Autodesk Inventor part; units mm, degrees
ref_plane "YZ Plane" through (0, 0, 0) normal (1, 0, 0) x (0, 1, 0)
ref_plane "XZ Plane" through (0, 0, 0) normal (0, 1, 0) x (-1, 0, 0)
ref_plane "XY Plane" through (0, 0, 0) normal (0, 0, 1) x (1, 0, 0)
sketch "Sketch1" plane through (0, 0, 0) normal (0, 0, 1) x (1, 0, 0)
  line L0 (0, 0) -> (9.525, 0)
  line L1 (9.525, 0) -> (9.525, 38.1)
  line L2 (9.525, 38.1) -> (31.75, 38.1)
  line L3 (0, 0) -> (0, 63.5) construction
  line L4 (0, 63.5) -> (-3.175, 63.5) construction
  line L5 (-3.175, 63.5) -> (31.75, 38.1)
  line L6 (0, 0) -> (0, 31.75)
  line L7 (4.7625, 0) -> (4.7625, 100.076) construction
  arc A0 (0, 31.75) -> (-3.175, 63.5) centre (-18.6849, 45.9153) ccw
  dimension "d0" = 9.525
  dimension "d1" = 38.1
  dimension "d2" = 22.225
  dimension "d3" = 63.5
  dimension "d4" = 3.175
  dimension "d5" = 4.7625
extrude "Extrusion1" add sketch "Sketch1" along normal blind 12.7
sketch "Sketch2" plane through (9.525, 0, 0) normal (1, 0, 0) x (0, 0, -1)
  line L0 (0, 0) -> (0, 38.1)
  line L1 (0, 0) -> (-12.7, 0)
  circle A0 centre (-6.35, 7.62) radius 3.3782
  circle A1 centre (-3.9688, 25.4) radius 1.5875
  circle A2 centre (-8.7312, 17.4625) radius 1.5875
  dimension "d8" = 6.7564
  dimension "d10" = 6.35
  dimension "d11" = 7.62
  dimension "d12" = 3.175
  dimension "d13" = 3.175
  dimension "d15" = 4.7625
  dimension "d16" = 3.9688
  dimension "d17" = 25.4
  dimension "d24" = 7.9375
extrude "Extrusion2" cut sketch "Sketch2" against normal blind 12.7
fillet "Fillet1" radius 3.175 1 edges at (9.525, 38.1, 6.35)
fillet "Fillet2" radius 0.3175 1 edges at (-3.175, 63.5, 6.35)
fillet "Fillet3" radius 0.3175 1 edges at (0, 31.75, 6.35)
fillet "Fillet4" radius 0.3175 1 edges at (31.75, 38.1, 6.35)
properties part number "Rebuild Puller Hook" material "Polycarbonate, Clear"
Can you work these out from the model? Positions are in its coordinate system, mm. A direction names the side the tool comes from. Give positions to 0.01 mm unless a question says otherwise; leave off trailing zeros. Order: outer loops, then holes, each group sorted by start corner. A loop starts at its lowest first (then second) coordinate and runs counter-clockwise, first axis right, second up. Notation, with made-up numbers: M 11,37.5 L 48,37.5 A35 cw 48,72.5 Z; hole C 74.5,79 d3. An arc over 180 degrees is marked long. Use one line per item in the form item = value. Start each with the question number.
Item 1: If we section it at B-B (y = 7.62): Write out the boundary of the cut face in (x, z) (3 decimals).
Item 2: For faces 1 (the flat face through (0, 16, 6)), 2 (the flat face through (9, 31, 12.7)), 3 (the flat face through (22, 38.1, 6)), which set-ups out of +Z, -Z, +X, -X, +Y, -Y let a thin tool reach every point of the face, with its end or its side?
Item 3: We'd pull the mould along Z, two halves only. Please class faces 4 (the flat face through (9, 31, 0)), 5 (the flat face through (9.525, 17, 6)), 6 (the cylindrical face through (4.829, 19.036, 8.938)): +Z half, -Z half, draft (parallel to the pull), parting line (faces both ways), or undercut.
Item 4: Will these pins go through, and if not, where does the flat tip stop? pin 1 Ø5 at (y, z) = (9, 4) entering from -X; pin 2 Ø4 at (x, z) = (8, 3.5) entering from +Y; pin 3 Ø4 at (x, z) = (4.5, 10) entering from +Y.
Item 5: If we section it at D-D (y = 25.4): Write out the boundary of the cut face in (x, z) (3 decimals).
Item 6: If I drill on line 1 along X through (y, z) = (4, 4.75) (3 decimals); line 2 along X through (y, z) = (33.5, 11.75) (3 decimals); line 3 along Y through (x, z) = (12.5, 5), over which ranges is the centre line in solid material (lowest first)?
Item 7: If we section it at C-C (z = 9): State how many separate pieces and enclosed holes the cut face has, then the cut area to 3 significant figures.
Outcome:
q1.outline = M 0,0 L 9.525,0 L 9.525,2.972 L 0,2.972 Z; M 0,9.728 L 9.525,9.728 L 9.525,12.7 L 0,12.7 Z
q2.face_1 = +Z, -Z, -X, -Y
q2.face_2 = +Z, +X, -X, +Y, -Y
q2.face_3 = +Z, -Z, +X, -Y
q3.face_4 = -Z half
q3.face_5 = draft
q3.face_6 = undercut
q4.pin_1 = 0
q4.pin_2 = 56.83
q4.pin_3 = 59.37
q5.outline = M 0,0 L 9.525,0 L 9.525,2.381 L 0,2.381 Z; M 0,5.556 L 9.525,5.556 L 9.525,12.7 L 0,12.7 Z
q6.line_1 = 0 to 9.525
q6.line_2 = 1.206 to 9.525
q6.line_3 = 38.09 to 52.1
q7.separate_pieces = 3
q7.enclosed_holes = 0
q7.area = 570 mm2
